Answer from the drawing. Dimensions are ordinates in mm from the lowest x, y and z of the part. Coordinates: 2 decimals unless noted, no trailing zeros. Write each loop counter-clockwise with the first axis right and the second up, starting at its lowest first coordinate (ties: lowest second). Pieces come first, ordered by that corner, then holes. Notation, with made-up numbers: (51, 20.25) - (87, 20.25) arc R6 ccw to (87, 29.25) - close; hole circle Ø8 at (36, 20.5). An arc over 180 degrees is marked (long way). Answer as a JSON object with one key per item and string values. Group by question number.
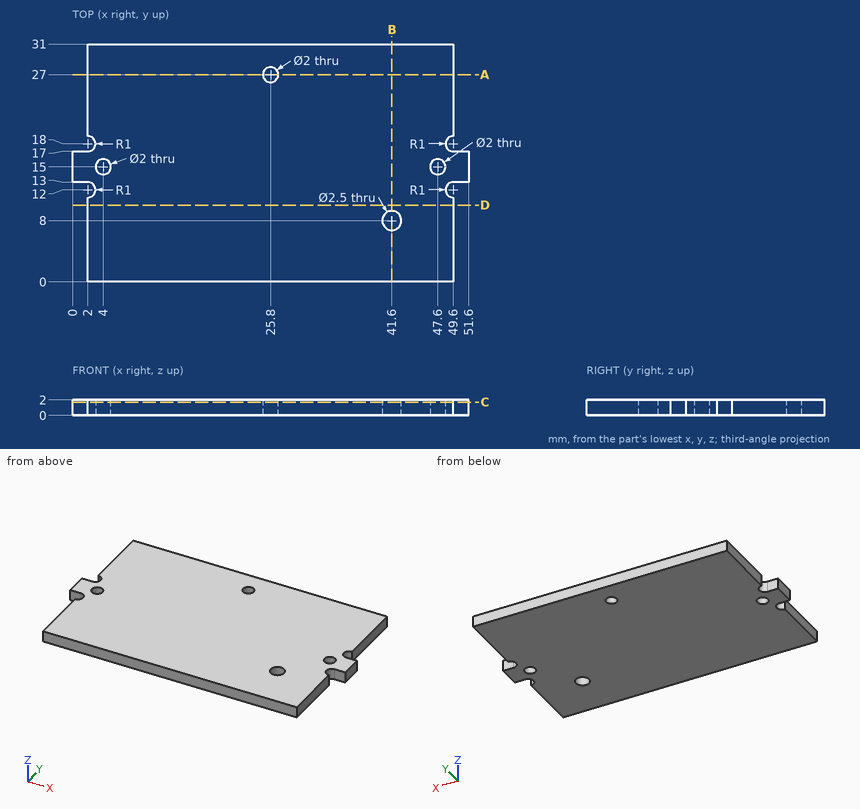
Q1. Section B-B on x = 41.6 is taken. Determine the outline of the cut face in (y, z).
Q2. Flat-ended cylindrical pins translate along their axes: pin 1 Ø1 at (y, z) = (3, 1) entering from -X; pin 2 Ø1 at (x, z) = (50.5, 1.5) entering from +Y; pin 3 Ø1 at (x, z) = (1, 1) entering from -Y. Find the tip coordinate at first contact, or state that the pin passes through.
Q3. Section A-A on y = 27 is taken. Determine the outline of the cut face in (x, z).
Q4. Section D-D on y = 10 is taken. Determine the outline of the cut face in (x, z), plus the area to 3 significant figures.
Q5. Consider L1, parallel to Y at x = 47.6, z = 1.3; L2, parallel to Y at x = 41.6, z = 0.4; L3, parallel to Y at x = 49, z = 0.7. Determine where each line is inside the solid, lowest interval first. Write a range as from..to.
Q6. Section C-C on z = 1.7 is taken. Determine the outline of the cut face in (x, y), plus the area to 3 significant figures.
Numbers:
{
 "1": {"outline": "(0, 0) - (6.75, 0) - (6.75, 2) - (0, 2) - close; (9.25, 0) - (31, 0) - (31, 2) - (9.25, 2) - close"},
 "2": {"pin 1": "stops at x = 2", "pin 2": "stops at y = 17", "pin 3": "stops at y = 13"},
 "3": {"outline": "(2, 0) - (24.8, 0) - (24.8, 2) - (2, 2) - close; (26.8, 0) - (49.6, 0) - (49.6, 2) - (26.8, 2) - close"},
 "4": {"outline": "(2, 0) - (49.6, 0) - (49.6, 2) - (2, 2) - close", "area": "95.2 mm²"},
 "5": {"L1": "y = 0..14, 16..31", "L2": "y = 0..6.75, 9.25..31", "L3": "y = 0..11.2, 12.8..17.2, 18.8..31"},
 "6": {"outline": "(0, 13) - (2, 13) arc R1 cw to (2, 11) - (2, 0) - (49.6, 0) - (49.6, 11) arc R1 cw to (49.6, 13) - (51.6, 13) - (51.6, 17) - (49.6, 17) arc R1 cw to (49.6, 19) - (49.6, 31) - (2, 31) - (2, 19) arc R1 cw to (2, 17) - (0, 17) - close; hole circle Ø2 at (4, 15); hole circle Ø2 at (25.8, 27); hole circle Ø2.5 at (41.6, 8); hole circle Ø2 at (47.6, 15)", "area": "1,470 mm²"}
}
